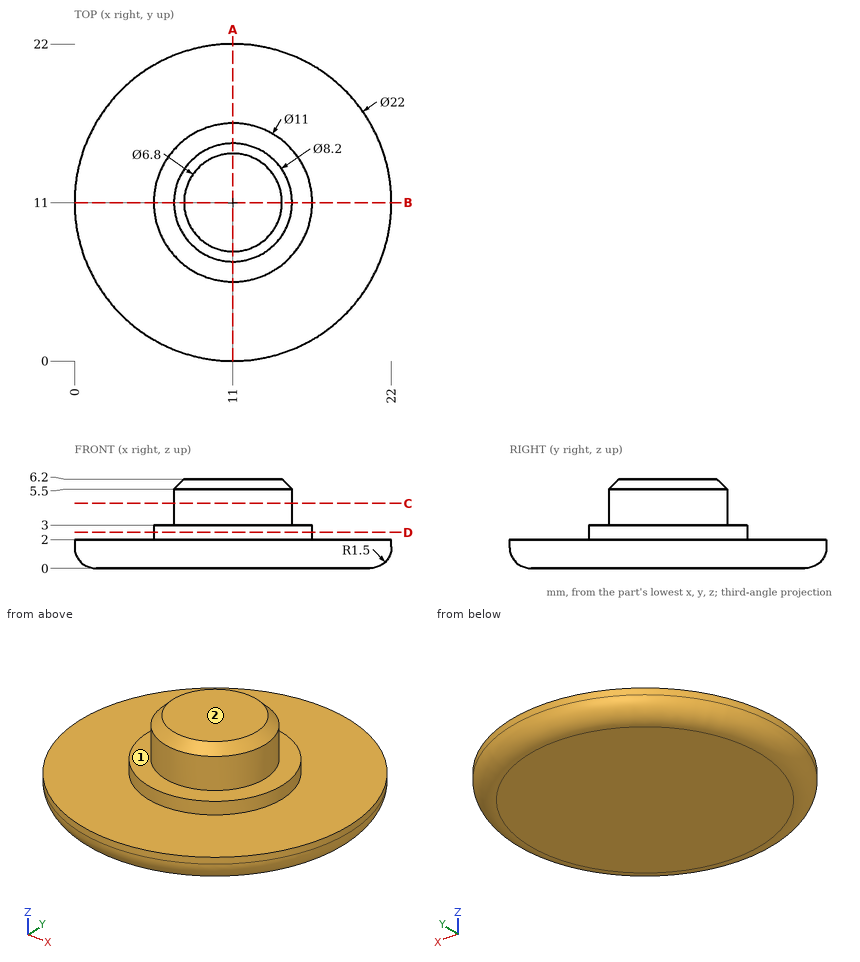
For this review, use the dimensioned drawing (mm, ordinates from the lowest corner) and the shaded views. A direction names the side the tool comes from. Coordinates: 2 decimals unless noted, no trailing zeros. Loops run counter-clockwise (first coordinate to the right, second up) from the corner with the lowest first, then second, coordinate; pieces in that order, holes last. Notation, with made-up numbers: (-33, 30.25) -> (2, 30.25) arc R21 ccw to (2, 62.25) -> close; hole circle Ø7 at (-11, 42). An arc over 180 degrees is marked (long way). Return JSON: item names as keys, results as strings. Group by question number.
(1) Consider section A-A, the plane x = 11. Give the boundary of the cut face in (y, z), plus the area to 3 significant figures.
(2) To check wall thickness, follow L1, parallel to Z at x = 3, y = 14.5; L2, parallel to Z at x = 8, y = 6.75; L3, parallel to X at y = 14.25, z = 1.75. State the ranges of each line that lie inside material, in increasing order.
(3) Consider section D-D, the plane z = 2.5. Give the boundary of the cut face in (x, y).
(4) For pin 1 Ø1.5 at (x, z) = (17, 1) entering from -Y; pin 2 Ø3 at (x, y) = (5, 16) entering from +Z; pin 3 Ø3 at (y, z) = (16, 2.5) entering from +X, all flat-tipped, find the tip position at first contact; note any pin that passes through.
(5) Tool access review of the marked faces 1 and 2: name each direction out of +Z, -Z, +X, -X, +Y, -Y from which nothing blocks a thin tool from reaching the whole face with its end or side.
(6) Consider section C-C, the plane z = 4.5. Give the boundary of the cut face in (x, y).
Results below:
{
 "1": {"outline": "(0, 1.5) arc R1.5 ccw to (1.5, 0) -> (20.5, 0) arc R1.5 ccw to (22, 1.5) -> (22, 2) -> (16.5, 2) -> (16.5, 3) -> (15.1, 3) -> (15.1, 5.5) -> (14.4, 6.2) -> (7.6, 6.2) -> (6.9, 5.5) -> (6.9, 3) -> (5.5, 3) -> (5.5, 2) -> (0, 2) -> close", "area": "79.8 mm2"},
 "2": {"L1": "z = 0 to 2", "L2": "z = 0 to 3", "L3": "x = 0.49 to 21.51"},
 "3": {"outline": "circle Ø11 at (11, 11)"},
 "4": {"pin 1": "stops at y = 1.38", "pin 2": "stops at z = 2", "pin 3": "stops at x = 21.4"},
 "5": {"face 1": "+Z", "face 2": "+Z, +X, -X, +Y, -Y"},
 "6": {"outline": "circle Ø8.2 at (11, 11)"}
}
